Here's the drawing with two shaded views (mm, measured from the low corner). I have some questions. A direction names the side the tool comes from. Coordinates: 2 decimals unless noted, no trailing zeros. Loops run counter-clockwise (first coordinate to the right, second up) from the corner with the lowest first, then second, coordinate; pieces in that order, holes last. Notation, with made-up numbers: (-18, 78) - (40, 78) arc R17 ccw to (40, 109) - close; hole circle Ø7 at (22, 57.25). An arc over 180 degrees is marked (long way). One line per item, written item: value. Start each with the question number.
(1) If we section it at B-B on z = 15.75: Write out the boundary of the cut face in (x, y), then the cut area to 3 significant figures.
(2) If we section it at C-C on y = 6.75: Write out the boundary of the cut face in (x, z).
(3) If we section it at A-A on x = 14.5: Write out the boundary of the cut face in (y, z), then the cut area to 3 significant figures.
(4) If we mould it in two halves opening along Y, with no side actions, what happens to the marked faces 3, 4 and 5? For each: pulls with the +Y half, pulls with the -Y half, needs draft (parallel to the pull), parting line crosses it, or undercut.
(5) I'm going to push flat-ended pins straight in: P1, Ø4, axis at x = 14, z = 7, coming from the +Y side; P2, Ø12, axis at x = 13, y = 10.5, coming from the +Z side. Where does each tip first touch, or does it pass through?
(6) On a 3-axis mill with a long thin cutter (end or side, diameter ignored), from which of +Z, -Z, +X, -X, +Y, -Y can I reach the whole of each face in a straight line? I mean the marked faces 1 and 2. Say none if no direction works.
(7) If I drill on line 1 along Y through (x, z) = (9.5, 19), over which ranges is the centre line in solid material (lowest first)? Write a range as from..to.
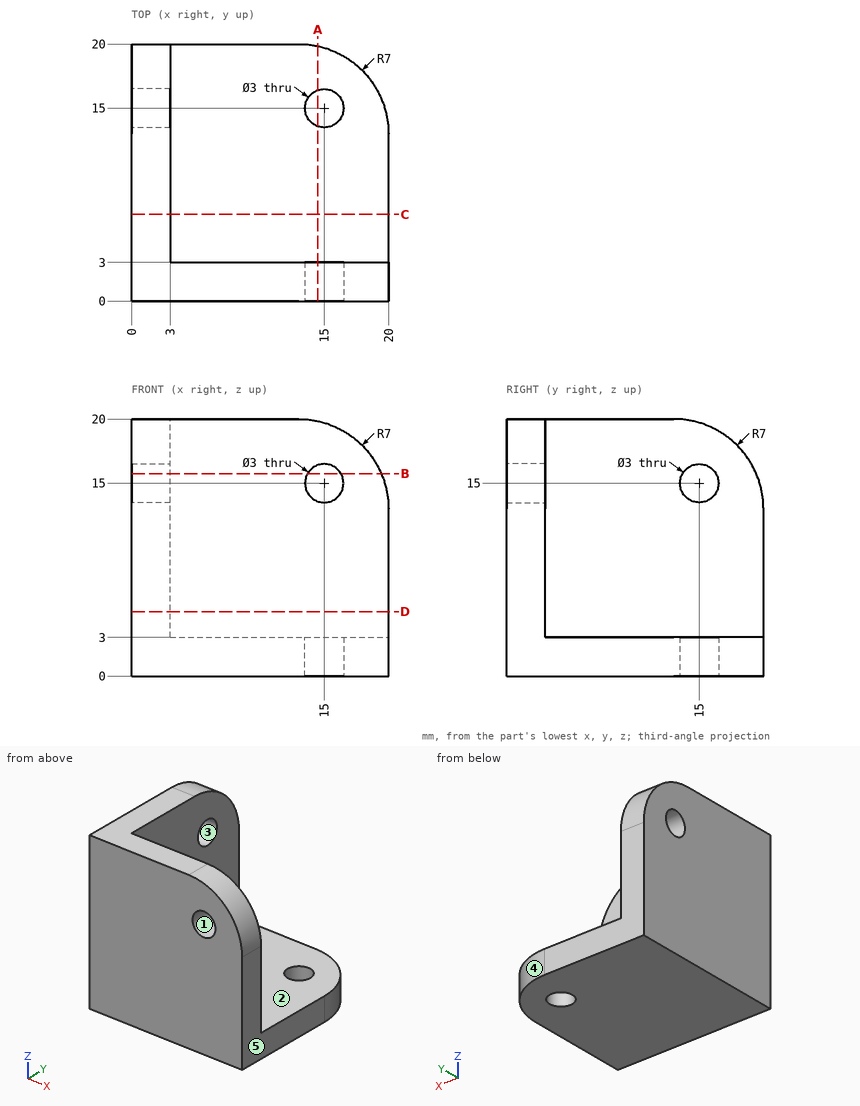
Values:
1. outline: (0, 0) - (13.7, 0) - (13.7, 3) - (3, 3) - (3, 13.7) - (0, 13.7) - close; (0, 16.3) - (3, 16.3) - (3, 19.44) - (0, 19.44) - close; (16.3, 0) - (19.44, 0) - (19.44, 3) - (16.3, 3) - close
1. area: 92.0 mm2
2. outline: (0, 0) - (20, 0) - (20, 3) - (3, 3) - (3, 20) - (0, 20) - close
3. outline: (0, 0) - (13.59, 0) - (13.59, 3) - (3, 3) - (3, 13.59) - (0, 13.59) - close; (0, 16.41) - (3, 16.41) - (3, 19.84) - (0, 19.84) - close; (16.41, 0) - (19.84, 0) - (19.84, 3) - (16.41, 3) - close
3. area: 93.1 mm2
4. face 3: undercut
4. face 4: pulls with the +Y half
4. face 5: needs draft
5. P1: stops at y = 3
5. P2: stops at z = 3
6. face 1: +Y, -Y
6. face 2: +Z, +X, +Y
7. line 1: y = 0..3
